Autodesk Fusion 360 part; units mm, degrees
sketch "Sketch1" plane through (0, 0, 0) normal (0, 0, 1) x (1, 0, 0)
  line L0 (0, 0) -> (5, 0) construction
  line L1 (5, 0) -> (7.0706, 7.7274) construction
  line L2 (5, 0) -> (13, 0) construction
  line L3 (5, 0) -> (7.0706, -7.7274) construction
  line L4 (5, 0) -> (13, 0) construction
  line L5 (0, 0) -> (-5, 0) construction
  line L6 (-5, 0) -> (-7.0706, 7.7274) construction
  line L7 (-5, 0) -> (0, 0) construction
  line L8 (-5, 0) -> (-7.0706, -7.7274) construction
  line L9 (-5, 0) -> (0, 0) construction
  line L10 (-7.0706, -7.7274) -> (7.0706, -7.7274) construction
  line L11 (-7.0706, 7.7274) -> (7.0706, 7.7274) construction
  line L12 (0, 0) -> (4.95, 0) construction
  line L13 (4.95, 0) -> (7.0076, 7.6791)
  line L14 (4.95, 0) -> (12.8, 0) construction
  line L15 (4.95, 0) -> (7.0076, -7.6791)
  line L16 (4.95, 0) -> (12.8, 0) construction
  line L17 (0, 0) -> (-4.95, 0) construction
  line L18 (-4.95, 0) -> (-7.0076, 7.6791)
  line L19 (-4.95, 0) -> (3, 0) construction
  line L20 (-7.0076, 7.6791) -> (7.0076, 7.6791)
  line L21 (-4.95, 0) -> (-7.0076, -7.6791)
  line L22 (-7.0076, -7.6791) -> (7.0076, -7.6791)
  dimension "d1" = 5
  dimension "d2" = 75
  dimension "d3" = 8
  dimension "d4" = 75
  dimension "d5" = 8
  dimension "d6" = 5
  dimension "d7" = 105
  dimension "d8" = 8
  dimension "d9" = 105
  dimension "d10" = 8
  dimension "d11" = 4.95
  dimension "d12" = 75
  dimension "d13" = 7.95
  dimension "d14" = 75
  dimension "d15" = 7.95
  dimension "d16" = 4.95
  dimension "d17" = 105
  dimension "d18" = 7.95
  dimension "d19" = 75
  dimension "d20" = 7.95
extrude "Extrude1" add sketch "Sketch1" along normal blind 3
Geometry: final body of the model. Coordinates: model frame, mm. A direction names the side the tool comes from. Coordinates: 2 decimals unless noted, no trailing zeros. Order: outer loops, then holes, each group sorted by start corner. A loop starts at its lowest first (then second) coordinate and runs counter-clockwise, first axis right, second up.
Item 1: Contact query for a flat-ended pin moving along its axis: P1, Ø1, axis at y = -5, z = 1.5, coming from the +X side. Output: stop coordinate, or through.
Answer:
P1: stops at x = 6.42
Item 2: Section query C-C (y = 2). Output: boundary loops of the cut face in (x, z).
Answer:
outline: (-5.49, 0) - (5.49, 0) - (5.49, 3) - (-5.49, 3) - close
Item 3: Access query for faces 4 (the face through (0, -7.679, 1)), 5 (the face through (5.964, -3.786, 1.479)), 6 (the face through (-5.964, -3.786, 1.479)). Directions: +Z, -Z, +X, -X, +Y, -Y. A direction counts if a zero-diameter tool reaches every point of the face in a straight line with its end or side. Return the directions, or none.
Answer:
face 4: +Z, -Z, +X, -X, -Y
face 5: +Z, -Z, +X
face 6: +Z, -Z, -X
Item 4: Section query D-D (y = 6). Output: boundary loops of the cut face in (x, z).
Answer:
outline: (-6.56, 0) - (6.56, 0) - (6.56, 3) - (-6.56, 3) - close
Item 5: Material intervals for line 1 along X through (y, z) = (3.25, 1.8); line 2 along X through (y, z) = (-1.75, 2.85), sorted ascending.
Answer:
line 1: x = -5.82 to 5.82
line 2: x = -5.42 to 5.42
Item 6: Section query A-A (z = 1.8). Output: boundary loops of the cut face in (x, y), then the cut area to 3 significant figures.
Answer:
outline: (-7.01, -7.68) - (7.01, -7.68) - (4.95, 0) - (7.01, 7.68) - (-7.01, 7.68) - (-4.95, 0) - close
area: 184 mm2
Item 7: Section query B-B (x = 6.25). Output: boundary loops of the cut face in (y, z).
Answer:
outline: (-7.68, 0) - (-4.85, 0) - (-4.85, 3) - (-7.68, 3) - close; (4.85, 0) - (7.68, 0) - (7.68, 3) - (4.85, 3) - close
Item 8: Draft query along Y for faces 1 (the face through (-5.964, 3.786, 1.479)), 2 (the face through (0, 7.679, 1)), 3 (the face through (0, 0, 3)). Return one class per face: released by +Y, released by -Y, zero draft, split by the parting line, or undercut.
Answer:
face 1: undercut
face 2: released by +Y
face 3: zero draft
